Print and shaded views of the part. All mm, measured from the part's lowest x, y and z. A direction names the side the tool comes from. Give positions to 0.01 mm unless a question says otherwise; leave off trailing zeros. Write each loop counter-clockwise with the first axis right and the second up, starting at its lowest first coordinate (ties: lowest second). Pieces come first, ordered by that corner, then holes. Notation, with made-up numbers: (-6, 38.5) -> (22, 38.5) arc R15 ccw to (22, 44.5) -> close; hole circle Ø9 at (-4, 29). An arc over 180 degrees is marked (long way). Put each result on its own line as item: value.
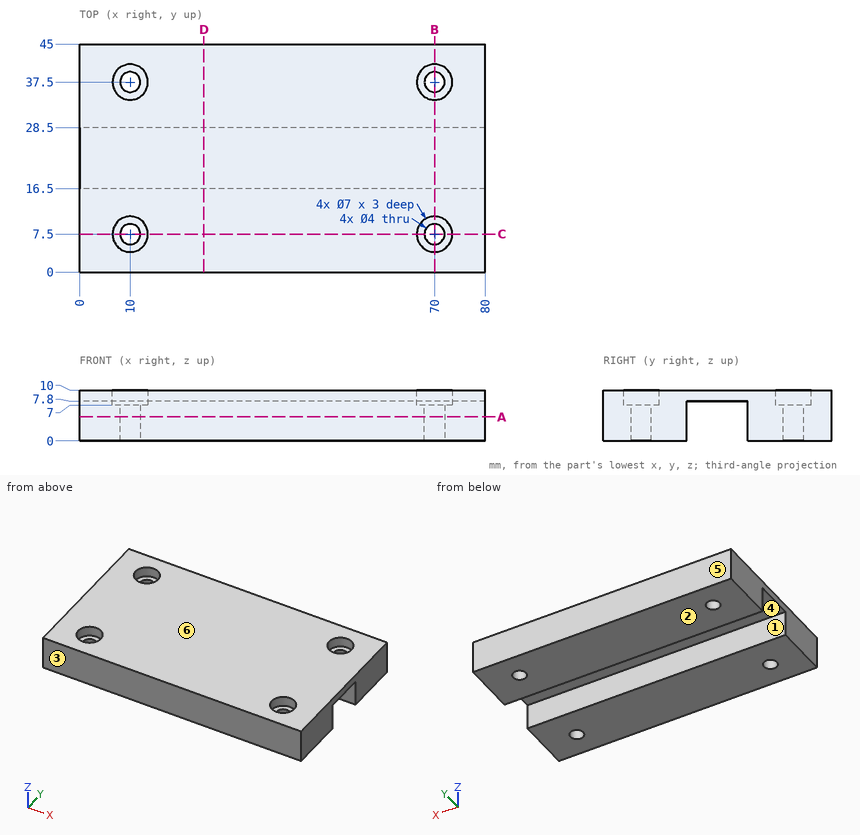
1) Slice it at C-C (y = 7.5). Write the cut outline in (x, z), plus the area to 3 significant figures.
Filled sheet:
outline: (0, 0) -> (8, 0) -> (8, 7) -> (6.5, 7) -> (6.5, 10) -> (0, 10) -> close; (12, 0) -> (68, 0) -> (68, 7) -> (66.5, 7) -> (66.5, 10) -> (13.5, 10) -> (13.5, 7) -> (12, 7) -> close; (72, 0) -> (80, 0) -> (80, 10) -> (73.5, 10) -> (73.5, 7) -> (72, 7) -> close
area: 702 mm2
2) Pull direction Y, two halves, no side cores. Call the marked faces 3, 4, 5 and 6: released by +Y, released by -Y, zero draft, split by the parting line, or undercut.
Filled sheet:
face 3: released by -Y
face 4: undercut
face 5: released by +Y
face 6: zero draft
3) Wall check: L1, parallel to Y at x = 70, z = 5.5; L2, parallel to Y at x = 10, z = 9.3; L3, parallel to Y at x = 13.5, z = 2.5. Give the ranges that are in metal, low to high.
Filled sheet:
L1: 0 to 5.5, 9.5 to 16.5, 28.5 to 35.5, 39.5 to 45
L2: 0 to 4, 11 to 34, 41 to 45
L3: 0 to 16.5, 28.5 to 45
4) Pin check, flat tips, straight feed: pin 1 (3.5 mm diameter, centred on x = 70, y = 7.5, fed in from -Z); pin 2 (2 mm diameter, centred on x = 9.5, y = 36.5, fed in from +Z). Stop position of each tip, or through.
Filled sheet:
pin 1: through
pin 2: z = 7
5) Slice it at A-A (z = 4.75). Write the cut outline in (x, y).
Filled sheet:
outline: (0, 0) -> (80, 0) -> (80, 16.5) -> (0, 16.5) -> close; (0, 28.5) -> (80, 28.5) -> (80, 45) -> (0, 45) -> close; hole circle Ø4 at (10, 7.5); hole circle Ø4 at (10, 37.5); hole circle Ø4 at (70, 7.5); hole circle Ø4 at (70, 37.5)
6) Slice it at B-B (x = 70). Write the cut outline in (y, z), plus the area to 3 significant figures.
Filled sheet:
outline: (0, 0) -> (5.5, 0) -> (5.5, 7) -> (4, 7) -> (4, 10) -> (0, 10) -> close; (9.5, 0) -> (16.5, 0) -> (16.5, 7.8) -> (28.5, 7.8) -> (28.5, 0) -> (35.5, 0) -> (35.5, 7) -> (34, 7) -> (34, 10) -> (11, 10) -> (11, 7) -> (9.5, 7) -> close; (39.5, 0) -> (45, 0) -> (45, 10) -> (41, 10) -> (41, 7) -> (39.5, 7) -> close
area: 258 mm2
7) Slice it at D-D (x = 24.5). Write the cut outline in (y, z), plus the area to 3 significant figures.
Filled sheet:
outline: (0, 0) -> (16.5, 0) -> (16.5, 7.8) -> (28.5, 7.8) -> (28.5, 0) -> (45, 0) -> (45, 10) -> (0, 10) -> close
area: 356 mm2
8) Tool access for the marked faces 1 and 2: list every direction of +Z, -Z, +X, -X, +Y, -Y with a clear straight run to the whole face (end or side of a thin tool).
Filled sheet:
face 1: -Z, +X, -X
face 2: -Z, +X, -X, +Y, -Y
